Geometry: final body of the model. Coordinates: model frame, mm. A direction names the side the tool comes from. Coordinates: 2 decimals unless noted, no trailing zeros. Write each loop counter-clockwise with the first axis right and the second up, starting at its lowest first coordinate (ties: lowest second). Pieces come first, ordered by that corner, then holes. Notation, with made-up numbers: (-21.5, 5.25) -> (-12.5, 5.25) arc R19 cw to (-12.5, 14.25) -> close; hole circle Ø7 at (21, 38.5). An arc over 180 degrees is marked (long way). One line per item, written item: value.
```python
from build123d import *

# Parameters (mm, degrees)
SKETCH1_W            = 26.5
SKETCH1_H            = 5.7
BOSS_EXTRUDE1_DEPTH  = 0.7
SKETCH1_3_W          = 30.9
SKETCH1_3_H          = 11.4
BOSS_EXTRUDE2_DEPTH  = 4.5
SKETCH1_4_W          = 29.3
SKETCH1_4_H          = 25.5
BOSS_EXTRUDE3_DEPTH  = 0.5
SKETCH1_5_W          = 15.7
SKETCH1_5_H          = 15.7
BOSS_EXTRUDE4_DEPTH  = 0.1
SKETCH1_7_W          = 17.5
SKETCH1_7_H          = 49.8
BOSS_EXTRUDE6_DEPTH  = 9.3
SKETCH1_8_W          = 26.6
SKETCH1_8_H          = 26.8
BOSS_EXTRUDE7_DEPTH  = 0.7
SKETCH1_10_W         = 2.5
SKETCH1_10_H         = 11.4
SKETCH1_10_W_2       = 4.7
SKETCH1_10_H_2       = 5.7
SKETCH1_10_W_3       = 3.3
SKETCH1_10_H_3       = 25.5
SKETCH1_10_W_4       = 6.35
SKETCH1_10_H_4       = 49.8
SKETCH1_10_W_5       = 2.75
BOSS_EXTRUDE8_DEPTH  = 14.8
SKETCH1_11_W         = 26.6
SKETCH1_11_H         = 26.8
SKETCH1_11_W_2       = 2.75
SKETCH1_11_H_2       = 49.8
SKETCH1_11_W_3       = 17.5
SKETCH1_11_W_4       = 6.35
SKETCH1_11_W_5       = 29.3
SKETCH1_11_H_3       = 25.5
SKETCH1_11_W_6       = 30.9
SKETCH1_11_H_4       = 11.4
SKETCH1_11_W_7       = 26.5
SKETCH1_11_H_5       = 5.7
SKETCH1_11_W_8       = 3.3
SKETCH1_11_W_9       = 4.7
SKETCH1_11_W_10      = 2.5
SKETCH1_11_W_11      = 15.7
SKETCH1_11_H_6       = 15.7
BOSS_EXTRUDE9_DEPTH  = 2
SKETCH1_12_W         = 39.85
SKETCH1_12_H         = 2
SKETCH1_12_W_2       = 4
BOSS_EXTRUDE10_DEPTH = 2
BOSS_EXTRUDE11_DEPTH = 27.2
SKETCH1_14_W         = 39.85
SKETCH1_14_H         = 2
SKETCH1_14_W_2       = 4
BOSS_EXTRUDE12_DEPTH = 14.8
BOSS_EXTRUDE13_DEPTH = 12.4
BOSS_EXTRUDE14_DEPTH = 32.7
BOSS_EXTRUDE15_DEPTH = 2
BOSS_EXTRUDE16_DEPTH = 16.2


with BuildPart() as part:
    # Sketch1 → Boss-Extrude1 (new body)
    with BuildSketch(Plane(origin=(0, 0, 0), x_dir=(1, 0, 0), z_dir=(0, 1, 0))):
        with Locations((-19.95, 11.55)):
            Rectangle(SKETCH1_W, SKETCH1_H)
    extrude(amount=BOSS_EXTRUDE1_DEPTH)



with BuildPart() as body_2:
    # Sketch1_3 → Boss-Extrude2 (new body)
    with BuildSketch(Plane(origin=(0, 0, 0), x_dir=(1, 0, 0), z_dir=(0, 1, 0))):
        with Locations((-19.95, -1)):
            Rectangle(SKETCH1_3_W, SKETCH1_3_H)
    extrude(amount=BOSS_EXTRUDE2_DEPTH)


with BuildPart() as body_3:
    # Sketch1_4 → Boss-Extrude3 (new body)
    with BuildSketch(Plane(origin=(0, 0, 0), x_dir=(1, 0, 0), z_dir=(0, 1, 0))):
        with Locations((-19.95, 31.15)):
            Rectangle(SKETCH1_4_W, SKETCH1_4_H)
    extrude(amount=BOSS_EXTRUDE3_DEPTH)


with BuildPart() as body_4:
    # Sketch1_5 → Boss-Extrude4 (new body)
    with BuildSketch(Plane(origin=(0, 0, 0), x_dir=(1, 0, 0), z_dir=(0, 1, 0))):
        with Locations((-30.05, -26.3)):
            Rectangle(SKETCH1_5_W, SKETCH1_5_H)
    extrude(amount=BOSS_EXTRUDE4_DEPTH)


with BuildPart() as body_5:
    # Sketch1_7 → Boss-Extrude6 (new body)
    with BuildSketch(Plane(origin=(0, 0, 0), x_dir=(1, 0, 0), z_dir=(0, 1, 0))):
        with Locations((17.1, -14.4)):
            Rectangle(SKETCH1_7_W, SKETCH1_7_H)
    extrude(amount=BOSS_EXTRUDE6_DEPTH)


with BuildPart() as body_6:
    # Sketch1_8 → Boss-Extrude7 (new body)
    with BuildSketch(Plane(origin=(0, 0, 0), x_dir=(1, 0, 0), z_dir=(0, 1, 0))):
        with Locations((15.3, 27.9)):
            Rectangle(SKETCH1_8_W, SKETCH1_8_H)
    extrude(amount=BOSS_EXTRUDE7_DEPTH)


with BuildPart() as part_1:
    add(part.part)

    add(body_2.part)  # Boss-Extrude8 merges body 2

    add(body_3.part)  # Boss-Extrude8 merges body 3

    add(body_4.part)  # Boss-Extrude8 merges body 4

    add(body_5.part)  # Boss-Extrude8 merges body 5

    add(body_6.part)  # Boss-Extrude8 merges body 6
    # Sketch1_10 → Boss-Extrude8 (add)
    with BuildSketch(Plane(origin=(0, 0, 0), x_dir=(1, 0, 0), z_dir=(0, 1, 0))):
        Polygon((-22.2, -41.9), (-18.2, -41.9), (-18.2, -10.7), (-22.2, -10.7), (-22.2, -18.45), (-22.2, -34.15), align=None)
        Polygon((-41.85, 51), (-41.85, -49), (-2, -49), (-2, -41.9), (-4.220803643, -41.9), (-18.2, -41.9), (-22.2, -41.9), (-32.120803643, -41.9), (-37.9, -41.9), (-37.9, -34.15), (-37.9, -18.45), (-37.9, -10.7), (-32.120803643, -10.7), (-22.2, -10.7), (-18.2, -10.7), (-4.220803643, -10.7), (-2, -10.7), (-2, -6.7), (-4.5, -6.7), (-35.4, -6.7), (-37.9, -6.7), (-37.9, 4.7), (-35.4, 4.7), (-4.5, 4.7), (-2, 4.7), (-2, 8.7), (-6.7, 8.7), (-33.2, 8.7), (-37.9, 8.7), (-37.9, 14.4), (-33.2, 14.4), (-6.7, 14.4), (-2, 14.4), (-2, 18.4), (-5.3, 18.4), (-34.6, 18.4), (-37.9, 18.4), (-37.9, 43.9), (-34.6, 43.9), (-5.3, 43.9), (-2, 43.9), (-2, 51), align=None)
        Polygon((-32.120803643, -41.9), (-22.2, -41.9), (-22.2, -34.15), (-37.9, -34.15), (-37.9, -41.9), align=None)
        Polygon((-22.2, -18.45), (-22.2, -10.7), (-32.120803643, -10.7), (-37.9, -10.7), (-37.9, -18.45), align=None)
        with Locations((-36.65, -1)):
            Rectangle(SKETCH1_10_W, SKETCH1_10_H)
        with Locations((-3.25, -1)):
            Rectangle(SKETCH1_10_W, SKETCH1_10_H)
        with Locations((-4.35, 11.55)):
            Rectangle(SKETCH1_10_W_2, SKETCH1_10_H_2)
        with Locations((-35.55, 11.55)):
            Rectangle(SKETCH1_10_W_2, SKETCH1_10_H_2)
        with Locations((-36.25, 31.15)):
            Rectangle(SKETCH1_10_W_3, SKETCH1_10_H_3)
        with Locations((-3.65, 31.15)):
            Rectangle(SKETCH1_10_W_3, SKETCH1_10_H_3)
        Polygon((-2, -41.9), (-2, -49), (2, -49), (2, -39.3), (2, 10.5), (2, 14.5), (2, 41.3), (2, 51), (-2, 51), (-2, 43.9), (-2, 18.4), (-2, 14.4), (-2, 8.7), (-2, 4.7), (-2, -6.7), (-2, -10.7), align=None)
        Polygon((2, -39.3), (2, -49), (41.85, -49), (41.85, 51), (2, 51), (2, 41.3), (28.6, 41.3), (28.6, 14.5), (2, 14.5), (2, 10.5), (8.35, 10.5), (25.85, 10.5), (28.6, 10.5), (28.6, -39.3), (25.85, -39.3), (8.35, -39.3), align=None)
        with Locations((5.175, -14.4)):
            Rectangle(SKETCH1_10_W_4, SKETCH1_10_H_4)
        with Locations((27.225, -14.4)):
            Rectangle(SKETCH1_10_W_5, SKETCH1_10_H_4)
    extrude(amount=BOSS_EXTRUDE8_DEPTH)

    # Sketch1_11 → Boss-Extrude9 (add)
    with BuildSketch(Plane(origin=(0, 0, 0), x_dir=(1, 0, 0), z_dir=(0, 1, 0))):
        Polygon((43.85, -51), (41.85, -51), (41.85, 51), (-41.85, 51), (-41.85, -51), (-43.85, -51), (-43.85, 53), (43.85, 53), align=None)
        Polygon((2, -39.3), (2, -49), (41.85, -49), (41.85, 51), (2, 51), (2, 41.3), (28.6, 41.3), (28.6, 14.5), (2, 14.5), (2, 10.5), (8.35, 10.5), (25.85, 10.5), (28.6, 10.5), (28.6, -39.3), (25.85, -39.3), (8.35, -39.3), align=None)
        with Locations((15.3, 27.9)):
            Rectangle(SKETCH1_11_W, SKETCH1_11_H)
        Polygon((-4.220803643, -41.9), (-2, -41.9), (-2, -10.7), (-4.220803643, -10.7), (-18.2, -10.7), (-18.2, -41.9), align=None)
        with Locations((27.225, -14.4)):
            Rectangle(SKETCH1_11_W_2, SKETCH1_11_H_2)
        with Locations((17.1, -14.4)):
            Rectangle(SKETCH1_11_W_3, SKETCH1_11_H_2)
        with Locations((5.175, -14.4)):
            Rectangle(SKETCH1_11_W_4, SKETCH1_11_H_2)
        Polygon((-2, -41.9), (-2, -49), (2, -49), (2, -39.3), (2, 10.5), (2, 14.5), (2, 41.3), (2, 51), (-2, 51), (-2, 43.9), (-2, 18.4), (-2, 14.4), (-2, 8.7), (-2, 4.7), (-2, -6.7), (-2, -10.7), align=None)
        Polygon((-41.85, 51), (-41.85, -49), (-2, -49), (-2, -41.9), (-4.220803643, -41.9), (-18.2, -41.9), (-22.2, -41.9), (-32.120803643, -41.9), (-37.9, -41.9), (-37.9, -34.15), (-37.9, -18.45), (-37.9, -10.7), (-32.120803643, -10.7), (-22.2, -10.7), (-18.2, -10.7), (-4.220803643, -10.7), (-2, -10.7), (-2, -6.7), (-4.5, -6.7), (-35.4, -6.7), (-37.9, -6.7), (-37.9, 4.7), (-35.4, 4.7), (-4.5, 4.7), (-2, 4.7), (-2, 8.7), (-6.7, 8.7), (-33.2, 8.7), (-37.9, 8.7), (-37.9, 14.4), (-33.2, 14.4), (-6.7, 14.4), (-2, 14.4), (-2, 18.4), (-5.3, 18.4), (-34.6, 18.4), (-37.9, 18.4), (-37.9, 43.9), (-34.6, 43.9), (-5.3, 43.9), (-2, 43.9), (-2, 51), align=None)
        with Locations((-19.95, 31.15)):
            Rectangle(SKETCH1_11_W_5, SKETCH1_11_H_3)
        with Locations((-19.95, -1)):
            Rectangle(SKETCH1_11_W_6, SKETCH1_11_H_4)
        with Locations((-19.95, 11.55)):
            Rectangle(SKETCH1_11_W_7, SKETCH1_11_H_5)
        with Locations((-3.65, 31.15)):
            Rectangle(SKETCH1_11_W_8, SKETCH1_11_H_3)
        with Locations((-36.25, 31.15)):
            Rectangle(SKETCH1_11_W_8, SKETCH1_11_H_3)
        with Locations((-35.55, 11.55)):
            Rectangle(SKETCH1_11_W_9, SKETCH1_11_H_5)
        with Locations((-4.35, 11.55)):
            Rectangle(SKETCH1_11_W_9, SKETCH1_11_H_5)
        with Locations((-3.25, -1)):
            Rectangle(SKETCH1_11_W_10, SKETCH1_11_H_4)
        with Locations((-36.65, -1)):
            Rectangle(SKETCH1_11_W_10, SKETCH1_11_H_4)
        with Locations((-30.05, -26.3)):
            Rectangle(SKETCH1_11_W_11, SKETCH1_11_H_6)
        Polygon((-22.2, -18.45), (-22.2, -10.7), (-32.120803643, -10.7), (-37.9, -10.7), (-37.9, -18.45), align=None)
        Polygon((-22.2, -41.9), (-18.2, -41.9), (-18.2, -10.7), (-22.2, -10.7), (-22.2, -18.45), (-22.2, -34.15), align=None)
        Polygon((-32.120803643, -41.9), (-22.2, -41.9), (-22.2, -34.15), (-37.9, -34.15), (-37.9, -41.9), align=None)
    extrude(amount=-BOSS_EXTRUDE9_DEPTH)

    # Sketch1_12 → Boss-Extrude10 (add)
    with BuildSketch(Plane(origin=(0, 0, 0), x_dir=(1, 0, 0), z_dir=(0, 1, 0))):
        with Locations((-21.925, -50)):
            Rectangle(SKETCH1_12_W, SKETCH1_12_H)
        with Locations((0, -50)):
            Rectangle(SKETCH1_12_W_2, SKETCH1_12_H)
        with Locations((21.925, -50)):
            Rectangle(SKETCH1_12_W, SKETCH1_12_H)
    extrude(amount=-BOSS_EXTRUDE10_DEPTH)

    # Sketch1_13 → Boss-Extrude11 (add)
    with BuildSketch(Plane(origin=(0, 0, 0), x_dir=(1, 0, 0), z_dir=(0, 1, 0))):
        Polygon((43.85, -51), (41.85, -51), (41.85, 51), (-41.85, 51), (-41.85, -51), (-43.85, -51), (-43.85, 53), (43.85, 53), align=None)
    extrude(amount=BOSS_EXTRUDE11_DEPTH)

    # Sketch1_14 → Boss-Extrude12 (add)
    with BuildSketch(Plane(origin=(0, 0, 0), x_dir=(1, 0, 0), z_dir=(0, 1, 0))):
        with Locations((-21.925, -50)):
            Rectangle(SKETCH1_14_W, SKETCH1_14_H)
        with Locations((0, -50)):
            Rectangle(SKETCH1_14_W_2, SKETCH1_14_H)
        with Locations((21.925, -50)):
            Rectangle(SKETCH1_14_W, SKETCH1_14_H)
    extrude(amount=BOSS_EXTRUDE12_DEPTH)

    # Sketch2 → Boss-Extrude13 (add)
    with BuildSketch(Plane(origin=(0, 14.8, 0), x_dir=(1, 0, 0), z_dir=(0, 1, 0))):
        Polygon((-39.85, -51), (-39.85, 49), (39.85, 49), (39.85, -51), (41.85, -51), (41.85, 51), (-41.85, 51), (-41.85, -51), align=None)
    extrude(amount=BOSS_EXTRUDE13_DEPTH)

    # Sketch1_15 → Boss-Extrude14 (add)
    with BuildSketch(Plane(origin=(0, 0, 0), x_dir=(1, 0, 0), z_dir=(0, 1, 0))):
        Polygon((43.85, -51), (41.85, -51), (41.85, 51), (-41.85, 51), (-41.85, -51), (-43.85, -51), (-43.85, 53), (43.85, 53), align=None)
    extrude(amount=BOSS_EXTRUDE14_DEPTH)

    # Sketch3 → Boss-Extrude15 (add)
    with BuildSketch(Plane(origin=(0, 32.7, 0), x_dir=(1, 0, 0), z_dir=(0, 1, 0))):
        Polygon((-41.85, -51), (-39.85, -51), (-39.85, 49), (39.85, 49), (39.85, -51), (41.85, -51), (41.85, 51), (-41.85, 51), align=None)
    extrude(amount=-BOSS_EXTRUDE15_DEPTH)

    # Sketch4 → Boss-Extrude16 (add)
    with BuildSketch(Plane(origin=(-18.2, 0, 0), x_dir=(0, 0, -1), z_dir=(1, 0, 0))):
        Polygon((-10.7, 10), (-10.7, 0), (-41.9, 0), align=None)
    extrude(amount=BOSS_EXTRUDE16_DEPTH)


solid = part_1.part
```
(1) Line query: line 1 (Z direction, x = -14, y = 11); line 2 (Z direction, x = -20, y = 13.5); line 3 (Z direction, x = -25, y = 9). Output: solid intervals per line, ascending. Write a range as [from, to].
Responses:
line 1: z = [-53, -43.9], [-18.4, -14.4], [-8.7, -4.7], [6.7, 10.7], [41.9, 51]
line 2: z = [-53, -43.9], [-18.4, -14.4], [-8.7, -4.7], [6.7, 51]
line 3: z = [-53, -43.9], [-18.4, -14.4], [-8.7, -4.7], [6.7, 18.45], [34.15, 51]
(2) Pull-direction query (Y, two-part tool) for faces 1 (the flat face through (-2, 9, 30)), 2 (the flat face through (-0.2, 27.2, -49.3)), 3 (the flat face through (-10.21, 4.93, 26.52)); classes: released by +Y, released by -Y, zero draft, split by the parting line, or undercut.
Responses:
face 1: zero draft
face 2: undercut
face 3: released by +Y
(3) Section B-B (y = 23). Return the cut outline in (x, z), then the cut area to 3 significant figures.
Responses:
outline: (-43.85, -53) -> (43.85, -53) -> (43.85, 51) -> (39.85, 51) -> (39.85, -49) -> (-39.85, -49) -> (-39.85, 51) -> (-43.85, 51) -> close
area: 1,150 mm2
(4) Section C-C (x = 18). Return the cut outline in (y, z), then the cut area to 3 significant figures.
Responses:
outline: (-2, -53) -> (32.7, -53) -> (32.7, -49) -> (30.7, -49) -> (30.7, -51) -> (27.2, -51) -> (27.2, -49) -> (14.8, -49) -> (14.8, -41.3) -> (0.7, -41.3) -> (0.7, -14.5) -> (14.8, -14.5) -> (14.8, -10.5) -> (9.3, -10.5) -> (9.3, 39.3) -> (14.8, 39.3) -> (14.8, 51) -> (-2, 51) -> close
area: 1,160 mm2
(5) Section A-A (y = 6). Return the cut outline in (x, z), then the cut area to 3 significant figures.
Responses:
outline: (-43.85, -53) -> (43.85, -53) -> (43.85, 51) -> (-43.85, 51) -> close; hole (-37.9, 18.45) -> (-22.2, 18.45) -> (-22.2, 34.15) -> (-37.9, 34.15) -> close; hole (-35.4, -4.7) -> (-4.5, -4.7) -> (-4.5, 6.7) -> (-35.4, 6.7) -> close; hole (-34.6, -43.9) -> (-5.3, -43.9) -> (-5.3, -18.4) -> (-34.6, -18.4) -> close; hole (-33.2, -14.4) -> (-6.7, -14.4) -> (-6.7, -8.7) -> (-33.2, -8.7) -> close; hole (-18.2, 23.18) -> (-2, 23.18) -> (-2, 41.9) -> (-18.2, 41.9) -> close; hole (2, -41.3) -> (28.6, -41.3) -> (28.6, -14.5) -> (2, -14.5) -> close
area: 6,610 mm2
(6) First-contact query: pin 1 (13 mm diameter, centred on x = -16.5, z = -35.5, fed in from +Y); pin 2 (5 mm diameter, centred on x = 8, z = 33.5, fed in from +Y); pin 3 (4 mm diameter, centred on x = 3.5, y = 29, fed in from +Z). Flat tips, straight axial feed; report the tip coordinate or a pass-through.
Responses:
pin 1: stops at y = 0.5
pin 2: stops at y = 14.8
pin 3: stops at z = -49
(7) Reachability of faces 4 (the flat face through (0, 32.7, -51)), 5 (the flat face through (-35.4, 10, 1)), 6 (the flat face through (-0.2, 30.7, -49.3)), 7 (the flat face through (39.85, 21, 0)) from +Z, -Z, +X, -X, +Y, -Y: full face, straight path, thin tool, end or side. Return the list, or none.
Responses:
face 4: +Z, -Z, +X, -X, +Y
face 5: +Y
face 6: +Z
face 7: +Z, +Y
(8) Section D-D (z = -22). Return the cut outline in (x, y).
Responses:
outline: (-43.85, -2) -> (43.85, -2) -> (43.85, 32.7) -> (39.85, 32.7) -> (39.85, 30.7) -> (41.85, 30.7) -> (41.85, 27.2) -> (39.85, 27.2) -> (39.85, 14.8) -> (28.6, 14.8) -> (28.6, 0.7) -> (2, 0.7) -> (2, 14.8) -> (-5.3, 14.8) -> (-5.3, 0.5) -> (-34.6, 0.5) -> (-34.6, 14.8) -> (-39.85, 14.8) -> (-39.85, 27.2) -> (-41.85, 27.2) -> (-41.85, 30.7) -> (-39.85, 30.7) -> (-39.85, 32.7) -> (-43.85, 32.7) -> close
